```python
from build123d import *

# Parameters (mm, degrees)
SKETCH007_W     = 140
SKETCH007_H     = 110
PAD003_DEPTH    = 20
SKETCH008_W     = 136
SKETCH008_H     = 106
POCKET004_DEPTH = 18
SKETCH009_R     = 4
SKETCH009_R_2   = 1.1
PAD004_DEPTH    = 3
SKETCH010_R     = 1.6
PAD005_DEPTH    = 13.6
SKETCH011_R     = 3
POCKET005_DEPTH = 10
SKETCH012_W     = 9.8
SKETCH012_H     = 13.6
POCKET006_DEPTH = 2
SKETCH014_W     = 17
SKETCH014_H     = 8
SKETCH014_W_2   = 8.5
PAD007_DEPTH    = 8.5
SKETCH015_W     = 52
SKETCH015_H     = 2
POCKET007_DEPTH = 3.9
FILLET_R        = 2
FILLET001_R     = 4
FILLET002_R     = 2


with BuildPart() as part:
    # Sketch007 → Pad003 (new body)
    with BuildSketch(Plane.XY):
        with Locations((50, -22)):
            Rectangle(SKETCH007_W, SKETCH007_H)
    extrude(amount=PAD003_DEPTH)

    # Sketch008 (on Face6 of Pad003) → Pocket004 (cut)
    with BuildSketch(Plane.XY.offset(20)):
        with Locations((50, -22)):
            Rectangle(SKETCH008_W, SKETCH008_H)
    extrude(amount=-POCKET004_DEPTH, mode=Mode.SUBTRACT)

    # Sketch009 (on Face11 of Pocket004) → Pad004 (join)
    with BuildSketch(Plane.XY.offset(2)):
        with Locations((39.5, -70)):
            Circle(SKETCH009_R)
        with Locations((39.5, -70)):
            Circle(SKETCH009_R_2, mode=Mode.SUBTRACT)
        with Locations((60.5, -70)):
            Circle(SKETCH009_R)
        with Locations((60.5, -70)):
            Circle(SKETCH009_R_2, mode=Mode.SUBTRACT)
    extrude(amount=PAD004_DEPTH)

    # Sketch010 (on Face11 of Pad004) → Pad005 (join)
    with BuildSketch(Plane.XY.offset(2)):
        with BuildLine():
            Line((110, -71), (110, -75))
            Line((110, -75), (118, -75))
            Line((118, -75), (118, -67))
            Line((118, -67), (114, -67))
            ThreePointArc((114, -67), (111.171573, -68.171573), (110, -71))
        make_face()
        with Locations((114, -71)):
            Circle(SKETCH010_R, mode=Mode.SUBTRACT)
        with BuildLine():
            Line((-14, -67), (-18, -67))
            Line((-18, -67), (-18, -75))
            Line((-18, -75), (-10, -75))
            Line((-10, -75), (-10, -71))
            ThreePointArc((-10, -71), (-11.171573, -68.171573), (-14, -67))
        make_face()
        with Locations((-14, -71)):
            Circle(SKETCH010_R, mode=Mode.SUBTRACT)
        with BuildLine():
            Line((-10, 27), (-10, 31))
            Line((-10, 31), (-18, 31))
            Line((-18, 31), (-18, 23))
            Line((-18, 23), (-14, 23))
            ThreePointArc((-14, 23), (-11.171573, 24.171573), (-10, 27))
        make_face()
        with Locations((-14, 27)):
            Circle(SKETCH010_R, mode=Mode.SUBTRACT)
        with BuildLine():
            Line((110, 27), (110, 31))
            Line((110, 31), (118, 31))
            Line((118, 31), (118, 23))
            Line((118, 23), (114, 23))
            ThreePointArc((110, 27), (111.171573, 24.171573), (114, 23))
        make_face()
        with Locations((114, 27)):
            Circle(SKETCH010_R, mode=Mode.SUBTRACT)
    extrude(amount=PAD005_DEPTH)

    # Sketch011 (on Face4 of Pad005) → Pocket005 (cut)
    with BuildSketch(Plane(origin=(0, 0, 0), x_dir=(1, 0, 0), z_dir=(0, 0, -1))):
        with Locations((-14, 71)):
            Circle(SKETCH011_R)
        with Locations((114, 71)):
            Circle(SKETCH011_R)
        with Locations((-14, -27)):
            Circle(SKETCH011_R)
        with Locations((114, -27)):
            Circle(SKETCH011_R)
    extrude(amount=-POCKET005_DEPTH, mode=Mode.SUBTRACT)

    # Sketch012 (on Face6 of Pocket005) → Pocket006 (cut)
    with BuildSketch(Plane.XZ.offset(77)):
        with Locations((50, 13.2)):
            Rectangle(SKETCH012_W, SKETCH012_H)
    extrude(amount=-POCKET006_DEPTH, mode=Mode.SUBTRACT)

    # Sketch014 (on Face24 of Pocket006) → Pad007 (join)
    with BuildSketch(Plane.XY.offset(2)):
        with Locations((50, -6.8)):
            Rectangle(SKETCH014_W, SKETCH014_H)
        with Locations((50, -56.8)):
            Rectangle(SKETCH014_W, SKETCH014_H)
        with Locations((-6.75, -6.8)):
            Rectangle(SKETCH014_W_2, SKETCH014_H)
        with Locations((106.75, -6.8)):
            Rectangle(SKETCH014_W_2, SKETCH014_H)
        with Locations((-6.75, -56.8)):
            Rectangle(SKETCH014_W_2, SKETCH014_H)
        with Locations((106.75, -56.8)):
            Rectangle(SKETCH014_W_2, SKETCH014_H)
    extrude(amount=PAD007_DEPTH)

    # Sketch015 (on Face74 of Pad007) → Pocket007 (cut)
    with BuildSketch(Plane.XY.offset(10.5)):
        with Locations((19.5, -6.8)):
            Rectangle(SKETCH015_W, SKETCH015_H)
        with Locations((19.5, -56.8)):
            Rectangle(SKETCH015_W, SKETCH015_H)
        with Locations((80.5, -6.8)):
            Rectangle(SKETCH015_W, SKETCH015_H)
        with Locations((80.5, -56.8)):
            Rectangle(SKETCH015_W, SKETCH015_H)
    extrude(amount=-POCKET007_DEPTH, mode=Mode.SUBTRACT)

    # Fillet
    fillet_edges = [part.edges().sort_by_distance(p)[0] for p in [
        (-18, -22, 2),
        (50, 31, 2),
        (118, -22, 2),
        (50, -75, 2),
        (-18, 31, 17.8),
        (118, 31, 17.8),
        (118, -75, 17.8),
        (-18, -75, 17.8),
        (-11, -10.8, 6.25),
        (-2.5, -10.8, 6.25),
        (41.5, -10.8, 6.25),
        (58.5, -10.8, 6.25),
        (102.5, -10.8, 6.25),
        (111, -10.8, 6.25),
        (-11, -60.8, 6.25),
        (-2.5, -60.8, 6.25),
        (41.5, -60.8, 6.25),
        (58.5, -60.8, 6.25),
        (102.5, -60.8, 6.25),
        (111, -60.8, 6.25),
        (-11, -52.8, 6.25),
        (-2.5, -52.8, 6.25),
        (41.5, -52.8, 6.25),
        (58.5, -52.8, 6.25),
        (102.5, -52.8, 6.25),
        (111, -52.8, 6.25),
        (-11, -2.8, 6.25),
        (-2.5, -2.8, 6.25),
        (41.5, -2.8, 6.25),
        (58.5, -2.8, 6.25),
        (102.5, -2.8, 6.25),
        (111, -2.8, 6.25),
    ]]
    fillet(fillet_edges, radius=FILLET_R)

    # Fillet001
    fillet001_edges = [part.edges().sort_by_distance(p)[0] for p in [
        (120, 33, 10),
        (120, -77, 10),
        (-20, 33, 10),
        (-20, -77, 10),
    ]]
    fillet(fillet001_edges, radius=FILLET001_R)

    # Fillet002
    fillet002_edges = [part.edges().sort_by_distance(p)[0] for p in [
        (-20, -22, 0),
    ]]
    fillet(fillet002_edges, radius=FILLET002_R)


with BuildPart() as part_1:
    # Body001 placement: moved
    add(part.part.moved(Location((0, 0, -23))))


solid = part_1.part
```
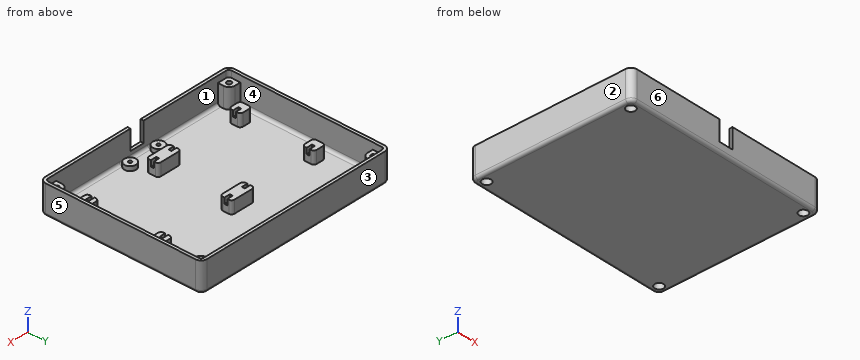
Build history of the part. All positions in model axes, mm. Face numbers are marked on the shaded views. A direction names the side the tool comes from. Give positions to 0.01 mm unless a question says otherwise; leave off trailing zeros. Order: outer loops, then holes, each group sorted by start corner. A loop starts at its lowest first (then second) coordinate and runs counter-clockwise, first axis right, second up. Notation, with made-up numbers: M 25.5,9 L 66.5,9 A30 ccw 66.5,33 Z; hole C 64.5,27 d4. An arc over 180 degrees is marked long. Write item = value, one per line. Start each with the question number.
(1) Pin check, flat tips, straight feed: pin 1 Ø2 at (x, z) = (51, -8.5) entering from -Y; pin 2 Ø9 at (x, y) = (-14, 28.5) entering from +Z; pin 3 Ø1 at (x, y) = (32, -5) entering from +Z; pin 4 Ø2.5 at (x, y) = (59.5, -71.5) entering from +Z. Stop position of each tip, or through.
(2) Two-plate mould, pull along Y, no slides. Class the marked faces 3, 4, 5 and 6: released by +Y, released by -Y, zero draft, split by the parting line, or undercut.
(3) Slice it at B-B on y = -31. Write the cut outline in (x, z).
(4) Probe L1, parallel to X at y = 27, z = -15; L2, parallel to X at y = 27, z = -10.4; L3, parallel to Y at x = 39.5, z = -18.75. List the from-to ranges inside material, lowest first. Write a range as [from, to].
(5) Slice it at A-A on x = 0.5. Write the cut outline in (y, z).
(6) Which spindle directions (+Z, -Z, +X, -X, +Y, -Y) get a long thin tool onto all of the face, cutting with end or side? Do the marked faces 1 and 2. Say none if no direction does.
Responses:
q1.pin_1 = 31
q1.pin_2 = -3
q1.pin_3 = -21
q1.pin_4 = -18
q2.face_3 = released by +Y
q2.face_4 = undercut
q2.face_5 = zero draft
q2.face_6 = released by -Y
q3.outline = M -20,-21 A2 ccw -18,-23 L 118,-23 A2 ccw 120,-21 L 120,-3 L 118,-3 L 118,-19 A2 cw 116,-21 L -16,-21 A2 cw -18,-19 L -18,-3 L -20,-3 Z
q4.L1 = [-20, -17], [-11, -10], [110, 111], [117, 120]
q4.L2 = [-20, -15.6], [-12.4, -10], [110, 112.4], [115.6, 120]
q4.L3 = [-77, -75], [-74, -71.1], [-68.9, -66], [31, 33]
q5.outline = M -77,-21 A2 ccw -75,-23 L 31,-23 A2 ccw 33,-21 L 33,-3 L 31,-3 L 31,-19 A2 cw 29,-21 L -73,-21 A2 cw -75,-19 L -75,-3 L -77,-3 Z
q6.face_1 = +Z
q6.face_2 = +Z, -Z, -X, +Y, -Y
